```python
from build123d import *

# Parameters (mm, degrees)
BOSS_EXTRUDE1_DEPTH        = 10
M2_5_START                 = 36.310160318
M2_5_CLEARANCE_SLOT1_DEPTH = 16


with BuildPart() as part:
    # Sketch1 → Boss-Extrude1 (new body)
    with BuildSketch(Plane.XY):
        with BuildLine():
            Line((0, 25.135160318), (0, 44.310160318))
            ThreePointArc((0, 44.310160318), (2.343145751, 49.967014567), (8, 52.310160318))
            Line((8, 52.310160318), (35.55, 52.310160318))
            ThreePointArc((35.55, 52.310160318), (36.964213562, 51.72437388), (37.55, 50.310160318))
            Line((37.55, 50.310160318), (37.55, 46.310160318))
            ThreePointArc((37.55, 46.310160318), (36.964213562, 44.895946756), (35.55, 44.310160318))
            Line((35.55, 44.310160318), (16, 44.310160318))
            ThreePointArc((16, 44.310160318), (10.343145751, 41.967014567), (8, 36.310160318))
            Line((8, 36.310160318), (8, 25.135160318))
            ThreePointArc((8, 25.135160318), (4, 21.135160318), (0, 25.135160318))
        make_face()
    extrude(amount=BOSS_EXTRUDE1_DEPTH)

    # M2.5 Clearance Slot1: read off the stored shape, not the designer's step
    # M2.5 Clearance Slot1 outline → M2.5 Clearance Slot1 (cut)
    with BuildSketch(Plane(origin=(0, 0, 0), x_dir=(1, 0, 0), z_dir=(0, 1, 0)).offset(M2_5_START)):
        with BuildLine():
            Line((12.5, -6.593666906), (27.5, -6.593666906))
            ThreePointArc((27.5, -6.593666906), (28.85, -5.243666906), (27.5, -3.893666906))
            Line((27.5, -3.893666906), (12.5, -3.893666906))
            ThreePointArc((12.5, -3.893666906), (11.15, -5.243666906), (12.5, -6.593666906))
        make_face()
    extrude(amount=M2_5_CLEARANCE_SLOT1_DEPTH, mode=Mode.SUBTRACT)


solid = part.part
```
For this review, take the finished solid that the model builds, in its own axes (mm). A direction names the side the tool comes from. Coordinates: 2 decimals unless noted, no trailing zeros. Order: outer loops, then holes, each group sorted by start corner. A loop starts at its lowest first (then second) coordinate and runs counter-clockwise, first axis right, second up. Notation, with made-up numbers: (-5.5, 50.5) -> (42.5, 50.5) arc R22 cw to (42.5, 58.5) -> close; hole circle Ø5 at (-17.5, 25.25). An arc over 180 degrees is marked (long way). Use CSV: the item, a comma, the result in double quotes. Start each with the question number.
Item 1: We need section D-D, the plane x = 34. Give the boundary of the cut face in (y, z).
Item 2: Wall thickness on probe 1 along Y at (x, z) = (12.5, 2.25); probe 2 along Y at (x, z) = (35.5, 4.75); probe 3 along X at (y, z) = (36, 7): over which ranges is each line inside the solid? List them lowest first.
Item 3: Draft analysis for pull direction Z (two halves, no side actions). For faces 1 (the face through (20, 48, 6.594)), 2 (the face through (22, 52.31, 3)), 3 (the face through (28.85, 48.25, 5.27)), 4 (the face through (11, 44, 0)), state which applies: pulls with the +Z half, pulls with the -Z half, needs draft (parallel to the pull), parting line crosses it, or undercut.
Item 4: For faces 5 (the face through (11.15, 47.42, 5.21)), 6 (the face through (28.1, 44.31, 3.8)), 7 (the face through (11, 44, 10)), list the 3-axis set-ups (+Z, -Z, +X, -X, +Y, -Y) from which the entire face can be reached by the end or side of a thin tool; tool diameter is ignored.
Item 5: We need section B-B, the plane y = 48. Give the boundary of the cut face in (x, z), then the cut area to 3 significant figures.
Item 6: We need section A-A, the plane x = 23.5. Give the boundary of the cut face in (y, z).
Item 7: We need section C-C, the plane z = 2.75. Give the boundary of the cut face in (x, y).
Item 8: Insertion check: pin 1 (6 mm diameter, centred on x = 20.5, y = 40, fed in from -Z). The pin has a flat end and moves straight along its axis. Give the tip position at first contact, or say it passes through.
Derived:
1,outline,"(44.31, 0) -> (52.31, 0) -> (52.31, 10) -> (44.31, 10) -> close"
2,probe 1,"y = 43.5 to 52.31"
2,probe 2,"y = 44.31 to 52.31"
2,probe 3,"x = 0 to 8"
3,face 1,"undercut"
3,face 2,"needs draft"
3,face 3,"undercut"
3,face 4,"pulls with the -Z half"
4,face 5,"+Y, -Y"
4,face 6,"+Z, -Z, +X, -Y"
4,face 7,"+Z, +X, -X, +Y, -Y"
5,outline,"(0.9, 0) -> (37.55, 0) -> (37.55, 10) -> (0.9, 10) -> close; hole (12.5, 3.89) -> (27.5, 3.89) arc R1.35 ccw to (27.5, 6.59) -> (12.5, 6.59) arc R1.35 ccw to start"
5,area,"320 mm^2"
6,outline,"(44.31, 0) -> (52.31, 0) -> (52.31, 3.89) -> (44.31, 3.89) -> close; (44.31, 6.59) -> (52.31, 6.59) -> (52.31, 10) -> (44.31, 10) -> close"
7,outline,"(0, 25.14) arc R4 ccw to (8, 25.14) -> (8, 36.31) arc R8 cw to (16, 44.31) -> (35.55, 44.31) arc R2 ccw to (37.55, 46.31) -> (37.55, 50.31) arc R2 ccw to (35.55, 52.31) -> (8, 52.31) arc R8 ccw to (0, 44.31) -> close"
8,pin 1,"passes through"
